Verification items for the finished model (mm, model axes). Give positions to 0.01 mm unless a question says otherwise; leave off trailing zeros. Loops run counter-clockwise (first coordinate to the right, second up) from the corner with the lowest first, then second, coordinate; pieces in that order, holes last. Notation, with made-up numbers: M 57.5,-34.75 L 76.5,-34.75 A24 cw 76.5,1.25 Z; hole C 51.25,-15.5 d4. An arc over 180 degrees is marked long. Use CSV: the item, a comma, the result in double quotes.
from build123d import *

# Parameters (mm, degrees)
SKETCH1_W           = 111
SKETCH1_H           = 111
BOSS_EXTRUDE1_DEPTH = 0.15
SKETCH2_W           = 13.5
SKETCH2_H           = 84.333333334
SKETCH2_W_2         = 84.333333334
SKETCH2_H_2         = 13.5
BOSS_EXTRUDE2_DEPTH = 1.3
FILLET1_R           = 2
FILLET2_R           = 1


with BuildPart() as part:
    # Sketch1 → Boss-Extrude1 (new, symmetric)
    with BuildSketch(Plane(origin=(0, 0, 0), x_dir=(1, 0, 0), z_dir=(0, 1, 0))):
        Rectangle(SKETCH1_W, SKETCH1_H)
    extrude(amount=BOSS_EXTRUDE1_DEPTH, both=True)

    # Sketch2 → Boss-Extrude2 (add)
    with BuildSketch(Plane.XZ.offset(0.15)):
        with Locations((-48.75, -3.5)):
            Rectangle(SKETCH2_W, SKETCH2_H)
        with Locations((3.5, -48.75)):
            Rectangle(SKETCH2_W_2, SKETCH2_H_2)
        with Locations((-3.5, 48.75)):
            Rectangle(SKETCH2_W_2, SKETCH2_H_2)
        with Locations((48.75, 3.5)):
            Rectangle(SKETCH2_W, SKETCH2_H)
    extrude(amount=BOSS_EXTRUDE2_DEPTH)

    # Fillet1
    fillet1_edges = [part.edges().sort_by_distance(p)[0] for p in [
        (45.666666667, -0.8, -55.5),
        (45.666666667, -0.8, -42),
        (-38.666666667, -0.8, -42),
        (-38.666666667, -0.8, -55.5),
        (-42, -0.8, -45.666666667),
        (-42, -0.8, 38.666666667),
        (-55.5, -0.8, 38.666666667),
        (-55.5, -0.8, -45.666666667),
        (-45.666666667, -0.8, 42),
        (38.666666667, -0.8, 42),
        (38.666666667, -0.8, 55.5),
        (-45.666666667, -0.8, 55.5),
        (42, -0.8, 45.666666667),
        (42, -0.8, -38.666666667),
        (55.5, -0.8, -38.666666667),
        (55.5, -0.8, 45.666666667),
    ]]
    fillet(fillet1_edges, radius=FILLET1_R)

    # Fillet2
    fillet2_edges = [part.edges().sort_by_distance(p)[0] for p in [
        (55.5, 0, 55.5),
        (-55.5, 0, 55.5),
        (-55.5, 0, -55.5),
        (55.5, 0, -55.5),
    ]]
    fillet(fillet2_edges, radius=FILLET2_R)


solid = part.part
(1) Scan lines: L1, parallel to X at y = -0.8, z = 12.5; L2, parallel to Z at x = 46, y = -0.95. Record each from-to range of solid material in increasing order. Write a range as from..to.
Calculated:
L1,"x = -55.5..-42, 42..55.5"
L2,"z = -38.67..45.67"
(2) Section check B-B on x = 3. Record the cut outline in (y, z), plus the area to 3 significant figures.
Calculated:
outline,"M -1.45,-55.5 L 0.15,-55.5 L 0.15,55.5 L -1.45,55.5 L -1.45,42 L -0.15,42 L -0.15,-42 L -1.45,-42 Z"
area,"68.4 mm²"
(3) Depth check by flat-ended pin: pin 1 Ø4 at (x, z) = (-2, -20) entering from -Y; pin 2 Ø0.6 at (x, y) = (50.5, -1) entering from -Z; pin 3 Ø0.6 at (x, y) = (-48, -0.5) entering from +Z. Enter the tip coordinate at first touch or a pass-through.
Calculated:
pin 1,"stops at y = -0.15"
pin 2,"stops at z = -38.67"
pin 3,"stops at z = 38.67"
(4) Section check D-D on x = 40.5. Record the cut outline in (y, z).
Calculated:
outline,"M -1.45,-55.5 L 0.15,-55.5 L 0.15,55.5 L -0.15,55.5 L -0.15,-42 L -1.45,-42 Z"
(5) Mould release check, pull along X, two halves, no side actions. Record for faces 1 (the flat face through (-1, -0.15, -1)), 2 (the flat face through (-1, 0.15, -1)): released by +X, released by -X, zero draft, split by the parting line, or undercut.
Calculated:
face 1,"undercut"
face 2,"zero draft"
(6) Section check A-A on y = -1. Count the separate pieces of the cut face and the enclosed holes in it, plus the area to 3 significant figures.
Calculated:
separate pieces,"4"
enclosed holes,"0"
area,"4,540 mm²"
(7) Section check C-C on z = -27.5. Record the cut outline in (x, y).
Calculated:
outline,"M -55.5,-1.45 L -42,-1.45 L -42,-0.15 L 42,-0.15 L 42,-1.45 L 55.5,-1.45 L 55.5,0.15 L -55.5,0.15 Z"
